from build123d import *

# Parameters (mm, degrees)
BOSS_EXTRUDE1_DEPTH  = 5
FILLET1_R            = 5
FILLET2_R            = 10
FILLET3_R            = 10
SKETCH3_R            = 1.5
CUT_EXTRUDE1_DEPTH   = 3.5
SKETCH5_W            = 12
SKETCH5_H            = 7
BOSS_EXTRUDE2_DEPTH  = 48
FILLET4_R            = 10
SKETCH6_W            = 4
SKETCH6_H            = 4
CUT_EXTRUDE2_DEPTH   = 30
FILLET4_OF_MIRROR1_R = 10


with BuildPart() as part:
    # Sketch1 → Boss-Extrude1 (new body)
    with BuildSketch(Plane(origin=(0, 0, 0), x_dir=(1, 0, 0), z_dir=(0, 1, 0))):
        Polygon((75.055534995, 0), (-54.848275573, 75), (-104.848275573, 75), (-104.848275573, -75), (-54.848275573, -75), align=None)
    extrude(amount=BOSS_EXTRUDE1_DEPTH)

    # Fillet1
    fillet1_edges = [part.edges().sort_by_distance(p)[0] for p in [
        (75.055534995, 2.5, 0),
    ]]
    fillet(fillet1_edges, radius=FILLET1_R)

    # Fillet2
    fillet2_edges = [part.edges().sort_by_distance(p)[0] for p in [
        (-54.848275573, 2.5, -75),
    ]]
    fillet(fillet2_edges, radius=FILLET2_R)

    # Fillet3
    fillet3_edges = [part.edges().sort_by_distance(p)[0] for p in [
        (-54.848275573, 2.5, 75),
    ]]
    fillet(fillet3_edges, radius=FILLET3_R)

    # Sketch3 → Cut-Extrude1 (cut)
    with BuildSketch(Plane(origin=(0, 5, 0), x_dir=(1, 0, 0), z_dir=(0, 1, 0))):
        with Locations(Location((-55.754465005, 0, 0), (0, 0, 270))):
            Circle(SKETCH3_R)
    extrude(amount=-CUT_EXTRUDE1_DEPTH, mode=Mode.SUBTRACT)

    # Sketch5 → Boss-Extrude2 (add)
    with BuildSketch(Plane.XZ):
        with Locations((-83.848275573, -31.5)):
            Rectangle(SKETCH5_W, SKETCH5_H)
    boss_extrude2 = extrude(amount=BOSS_EXTRUDE2_DEPTH)

    # Fillet4
    fillet4_edges = [part.edges().sort_by_distance(p)[0] for p in [
        (-89.848275573, 0, -31.5),
        (-83.848275573, 0, -35),
        (-77.848275573, 0, -31.5),
        (-83.848275573, 0, -28),
    ]]
    fillet(fillet4_edges, radius=FILLET4_R)

    # Sketch6 → Cut-Extrude2 (cut)
    with BuildSketch(Plane.XZ.offset(48)):
        with Locations((-83.848275573, -29)):
            Rectangle(SKETCH6_W, SKETCH6_H)
    cut_extrude2 = extrude(amount=-CUT_EXTRUDE2_DEPTH, mode=Mode.SUBTRACT)

    # Mirror1: Boss-Extrude2, Cut-Extrude2 across plane
    add(boss_extrude2.mirror(Plane.XY))
    add(cut_extrude2.mirror(Plane.XY), mode=Mode.SUBTRACT)

    # Fillet4 of Mirror1
    fillet4_of_mirror1_edges = [part.edges().sort_by_distance(p)[0] for p in [
        (-89.848275573, 0, 31.5),
        (-83.848275573, 0, 35),
        (-77.848275573, 0, 31.5),
        (-83.848275573, 0, 28),
    ]]
    fillet(fillet4_of_mirror1_edges, radius=FILLET4_OF_MIRROR1_R)


solid = part.part
Design review of the part built by this model. Coordinates are the model's own, in mm. A direction names the side the tool comes from. Coordinates: 2 decimals unless noted, no trailing zeros. Order: outer loops, then holes, each group sorted by start corner. A loop starts at its lowest first (then second) coordinate and runs counter-clockwise, first axis right, second up.
Item 1: For pin 1 Ø7.5 at (y, z) = (-26, -32) entering from -X; pin 2 Ø6 at (x, y) = (-83, -26.5) entering from +Z; pin 3 Ø3 at (x, z) = (-70, -16.5) entering from -Y, all flat-tipped, find the tip position at first contact; note any pin that passes through.
Item 2: Take a section at A-A, the plane y = -20. Write out the cut boundary in (x, z).
Item 3: For line 1 (X direction, y = -25, z = 29); line 2 (X direction, y = 2.75, z = 0); line 3 (Z direction, x = -78.5, y = -28), list the stretches that pass through material, from the lowest coordinate up.
Item 4: Take a section at D-D, the plane x = -32. Write out the cut boundary in (y, z), then the cut area to 3 significant figures.
Item 5: The part is to be moulded in two halves that separate along Z. For faces 1 (the flat face through (-84, -29, 35)), 2 (the flat face through (-84, -33, 31)), 3 (the flat face through (-83.9, -48, 31.5)), say which applies: pulls with the +Z half, pulls with the -Z half, needs draft (parallel to the pull), parting line crosses it, or undercut.
Item 6: For faces 4 (the flat face through (-87, -29, -28)), 5 (the flat face through (-77.848, -29, 32)), 6 (the flat face through (-84, -29, -35)), list the 3-axis set-ups (+Z, -Z, +X, -X, +Y, -Y) from which the entire face can be reached by the end or side of a thin tool; tool diameter is ignored.
Item 7: Take a section at B-B, the plane y = -5. Write out the cut boundary in (x, z).
Item 8: Take a section at C-C, the plane z = -24.5. Write out the cut boundary in (x, y), then the cut area to 3 significant figures.
The answers:
1. pin 1: stops at x = -89.85
1. pin 2: stops at z = 35
1. pin 3: stops at y = 0
2. outline: (-89.85, -35) - (-77.85, -35) - (-77.85, -28) - (-81.85, -28) - (-81.85, -31) - (-85.85, -31) - (-85.85, -28) - (-89.85, -28) - close; (-89.85, 28) - (-85.85, 28) - (-85.85, 31) - (-81.85, 31) - (-81.85, 28) - (-77.85, 28) - (-77.85, 35) - (-89.85, 35) - close
3. line 1: x = -89.85 to -85.85, -81.85 to -77.85
3. line 2: x = -104.85 to -57.25, -54.25 to 70.06
3. line 3: z = -35 to -28, 28 to 35
4. outline: (0, -61.81) - (5, -61.81) - (5, 61.81) - (0, 61.81) - close
4. area: 618 mm2
5. face 1: pulls with the +Z half
5. face 2: undercut
5. face 3: needs draft
6. face 4: +X, -X, -Y
6. face 5: +Z, -Z, +X, -Y
6. face 6: -Z, +X, -X, -Y
7. outline: (-91.19, -36.34) - (-76.51, -36.34) - (-76.51, -26.66) - (-91.19, -26.66) - close; (-91.19, 26.66) - (-76.51, 26.66) - (-76.51, 36.34) - (-91.19, 36.34) - close
8. outline: (-104.85, 0) - (-99.85, 0) arc R10 cw to (-93.35, -2.4) - (-74.35, -2.4) arc R10 cw to (-67.85, 0) - (32.62, 0) - (32.62, 5) - (-104.85, 5) - close
8. area: 743 mm2
